The model under review builds one solid part; all positions refer to its coordinate system, in mm. A direction names the side the tool comes from. Round coordinates to 2 decimals unless told otherwise and drop trailing zeros. Loops run counter-clockwise (first coordinate to the right, second up) from the corner with the lowest first, then second, coordinate; pieces in that order, holes last. Notation, with made-up numbers: M 3.25,30 L 55.25,30 A19 cw 55.25,54 Z; hole C 78,-1 d3. An arc over 180 degrees is marked long. Answer in a Markdown table with one row per item. Add a question column.
from build123d import *

# Parameters (mm, degrees)
EXTRUDE_THIN1_DEPTH                       = 20
SKETCH2_R                                 = 20
BOSS_EXTRUDE1_DEPTH                       = 42
FILLET1_RADIUS                            = 20
FILLET1_LENGTH                            = 12
SKETCH3_R                                 = 15
BOSS_EXTRUDE2_DEPTH                       = 21
SKETCH4_R                                 = 11.5
BOSS_EXTRUDE3_DEPTH                       = 10
CUT_EXTRUDE1_START                        = -10
CUT_EXTRUDE1_DEPTH                        = 10
F_18_0_18_DIAMETER_HOLE1_D                = 18
CBORE_FOR_M8_HEX_HEAD_BOLT1_OUTLINE_R     = 4.5
CBORE_FOR_M8_HEX_HEAD_BOLT1_DEPTH         = 43
CBORE_FOR_M8_HEX_HEAD_BOLT1_2_OUTLINE_R   = 9.005
CBORE_FOR_M8_HEX_HEAD_BOLT1_2_OUTLINE_R_2 = 4.5
CBORE_FOR_M8_HEX_HEAD_BOLT1_2_DEPTH       = 5.68
FILLET2_R                                 = 2


# Read off the part's stored shape, not the designer's step: CBORE for M8 Hex Head Bolt1
with BuildPart() as part:
    # Sketch1 → Extrude-Thin1 (new, symmetric)
    with BuildSketch(Plane(origin=(0, 0, 0), x_dir=(0, 0, -1), z_dir=(1, 0, 0))):
        with BuildLine():
            Line((0, 0), (52, 0))
            ThreePointArc((52, 0), (64.727922061, 5.272077939), (70, 18))
            Line((70, 18), (70, 57))
            ThreePointArc((70, 57), (64.727922061, 69.727922061), (52, 75))
            Line((52, 75), (-30, 75))
            Line((-30, 75), (-30, 63))
            Line((-30, 63), (52, 63))
            ThreePointArc((52, 63), (56.242640687, 61.242640687), (58, 57))
            Line((58, 57), (58, 18))
            ThreePointArc((58, 18), (56.242640687, 13.757359313), (52, 12))
            Line((52, 12), (0, 12))
            Line((0, 12), (0, 0))
        make_face()
    extrude(amount=EXTRUDE_THIN1_DEPTH, both=True)

    # Sketch2 → Boss-Extrude1 (add)
    with BuildSketch(Plane.XZ.offset(-63)):
        with Locations(Location((0, 30, 0), (0, 0, 270))):
            Circle(SKETCH2_R)
    extrude(amount=-BOSS_EXTRUDE1_DEPTH)

    # Fillet1: full round fillet: the end face becomes a half cylinder, R = half its width
    fillet1_face = Plane((0, 6, 0), x_dir=(0, -1, 0), z_dir=(0, 0, 1))  # on the end face: x along it, z out of the body
    fillet1_slab = fillet1_face.offset(-FILLET1_RADIUS / 2) * Box(FILLET1_LENGTH, 2 * FILLET1_RADIUS, FILLET1_RADIUS, mode=Mode.PRIVATE)  # the body's end, R deep
    fillet1_round = Plane((0, 6, -20), x_dir=(0, 0, 1), z_dir=(0, -1, 0)) * Cylinder(FILLET1_RADIUS, FILLET1_LENGTH, mode=Mode.PRIVATE)  # its axis R under the face
    add(fillet1_slab - fillet1_round, mode=Mode.SUBTRACT)

    # Sketch3 → Boss-Extrude2 (add)
    with BuildSketch(Plane(origin=(0, 12, 0), x_dir=(1, 0, 0), z_dir=(0, 1, 0))):
        with Locations(Location((0, 20, 0), (0, 0, 90))):
            Circle(SKETCH3_R)
    extrude(amount=BOSS_EXTRUDE2_DEPTH)

    # Sketch4 → Boss-Extrude3 (add)
    with BuildSketch(Plane(origin=(0, 33, 0), x_dir=(1, 0, 0), z_dir=(0, 1, 0))):
        with Locations(Location((0, 20, 0), (0, 0, 90))):
            Circle(SKETCH4_R)
    extrude(amount=BOSS_EXTRUDE3_DEPTH)

    # Sketch5 → Cut-Extrude1 (cut)
    with BuildSketch(Plane(origin=(0, 105, 0), x_dir=(1, 0, 0), z_dir=(0, 1, 0)).offset(CUT_EXTRUDE1_START)):
        with BuildLine():
            Line((-19.078784028, -24), (19.078784028, -24))
            ThreePointArc((19.078784028, -24), (0, -10), (-19.078784028, -24))
        make_face()
        with BuildLine():
            Line((-19.078784028, -36), (19.078784028, -36))
            ThreePointArc((19.078784028, -36), (0, -50), (-19.078784028, -36))
        make_face()
    extrude(amount=CUT_EXTRUDE1_DEPTH, mode=Mode.SUBTRACT)

    # Ø18.0 (18) Diameter Hole1 (through all)
    with Locations(Plane(origin=(0, 63, 0), x_dir=(-1, 0, 0), z_dir=(0, -1, 0))):
        with Locations((0, -30)):
            Hole(F_18_0_18_DIAMETER_HOLE1_D / 2)

    # CBORE for M8 Hex Head Bolt1 outline → CBORE for M8 Hex Head Bolt1 (cut)
    with BuildSketch(Plane(origin=(0, 0, 0), x_dir=(1, 0, 0), z_dir=(0, 1, 0))):
        with Locations((0, 20)):
            Circle(CBORE_FOR_M8_HEX_HEAD_BOLT1_OUTLINE_R)
    extrude(amount=CBORE_FOR_M8_HEX_HEAD_BOLT1_DEPTH, mode=Mode.SUBTRACT)

    # CBORE for M8 Hex Head Bolt1 2 outline → CBORE for M8 Hex Head Bolt1 2 (cut)
    with BuildSketch(Plane(origin=(0, 0, 0), x_dir=(1, 0, 0), z_dir=(0, 1, 0))):
        with Locations((0, 20)):
            Circle(CBORE_FOR_M8_HEX_HEAD_BOLT1_2_OUTLINE_R)
        with Locations((0, 20)):
            Circle(CBORE_FOR_M8_HEX_HEAD_BOLT1_2_OUTLINE_R_2, mode=Mode.SUBTRACT)
    extrude(amount=CBORE_FOR_M8_HEX_HEAD_BOLT1_2_DEPTH, mode=Mode.SUBTRACT)

    # Fillet2
    # the kernel refuses this fillet: 2 mm, written as the material it takes off along each edge
    with BuildSketch(Plane(origin=(20, 63, 30), x_dir=(0, 1, 0), z_dir=(0, 0, -1))) as fillet2_piece_1:
        with BuildLine():
            CenterArc((FILLET2_R, -FILLET2_R), FILLET2_R, 90, 90)
            Line((0, -FILLET2_R), (0, 0))
            Line((0, 0), (FILLET2_R, 0))
        make_face()
    extrude(amount=82, mode=Mode.SUBTRACT)
    with BuildSketch(Plane(origin=(-20, 18, -52), x_dir=(0, 0, -1), z_dir=(0, 1, 0))) as fillet2_piece_2:
        with BuildLine():
            CenterArc((6 + FILLET2_R, -FILLET2_R), FILLET2_R, 90, 90)
            Line((6 + FILLET2_R, 0), (6, 0))
            Line((6, 0), (6, -FILLET2_R))
        make_face()
    revolve(axis=Axis((-20, 18, -52), (-1, 0, 0)), revolution_arc=90, mode=Mode.SUBTRACT)
    with BuildSketch(Plane(origin=(-20, 57, -58), x_dir=(0, 0, -1), z_dir=(0, -1, 0)), Plane(origin=(-20, 18, -70), x_dir=(0, 0, 1), z_dir=(0, 1, 0))) as fillet2_piece_3:
        with BuildLine():
            CenterArc((FILLET2_R, FILLET2_R), FILLET2_R, 180, 90)
            Line((0, FILLET2_R), (0, 0))
            Line((0, 0), (FILLET2_R, 0))
        make_face()
    extrude(amount=39, mode=Mode.SUBTRACT)
    with BuildSketch(Plane(origin=(-20, 57, -52), x_dir=(0, 1, 0), z_dir=(0, 0, 1))) as fillet2_piece_4:
        with BuildLine():
            CenterArc((6 + FILLET2_R, -FILLET2_R), FILLET2_R, 90, 90)
            Line((6, -FILLET2_R), (6, 0))
            Line((6, 0), (6 + FILLET2_R, 0))
        make_face()
    revolve(axis=Axis((-20, 57, -52), (-1, 0, 0)), revolution_arc=90, mode=Mode.SUBTRACT)
    with BuildSketch(Plane(origin=(-20, 63, 30), x_dir=(0, 1, 0), z_dir=(0, 0, -1))) as fillet2_piece_5:
        with BuildLine():
            CenterArc((FILLET2_R, FILLET2_R), FILLET2_R, 180, 90)
            Line((0, FILLET2_R), (0, 0))
            Line((0, 0), (FILLET2_R, 0))
        make_face()
    extrude(amount=82, mode=Mode.SUBTRACT)
    with BuildSketch(Plane(origin=(-20, 75, -52), x_dir=(0, -1, 0), z_dir=(0, 0, 1))) as fillet2_piece_6_section:
        with BuildLine():
            CenterArc((FILLET2_R, FILLET2_R), FILLET2_R, 180, 90)
            Line((0, FILLET2_R), (0, 0))
            Line((0, 0), (FILLET2_R, 0))
        make_face()
    fillet2_piece_6 = extrude(amount=87, mode=Mode.PRIVATE)
    fillet2_piece_6 = fillet2_piece_6 - Plane(origin=(0, 74.534164155, 30), x_dir=(0, 0, -1), z_dir=(0, -1, 0)) * Cylinder(20, 182, mode=Mode.PRIVATE)
    add(fillet2_piece_6, mode=Mode.SUBTRACT)
    with BuildSketch(Plane(origin=(20, 57, -52), x_dir=(0, 1, 0), z_dir=(0, 0, 1))) as fillet2_piece_7:
        with BuildLine():
            CenterArc((6 + FILLET2_R, FILLET2_R), FILLET2_R, 180, 90)
            Line((6, FILLET2_R), (6, 0))
            Line((6, 0), (6 + FILLET2_R, 0))
        make_face()
    revolve(axis=Axis((20, 57, -52), (-1, 0, 0)), revolution_arc=90, mode=Mode.SUBTRACT)
    with BuildSketch(Plane(origin=(20, 57, -58), x_dir=(0, 0, -1), z_dir=(0, -1, 0)), Plane(origin=(20, 18, -70), x_dir=(0, 0, 1), z_dir=(0, 1, 0))) as fillet2_piece_8:
        with BuildLine():
            CenterArc((FILLET2_R, -FILLET2_R), FILLET2_R, 90, 90)
            Line((0, -FILLET2_R), (0, 0))
            Line((0, 0), (FILLET2_R, 0))
        make_face()
    extrude(amount=39, mode=Mode.SUBTRACT)
    with BuildSketch(Plane(origin=(20, 18, -52), x_dir=(0, 0, -1), z_dir=(0, 1, 0))) as fillet2_piece_9:
        with BuildLine():
            CenterArc((6 + FILLET2_R, FILLET2_R), FILLET2_R, 180, 90)
            Line((6 + FILLET2_R, 0), (6, 0))
            Line((6, 0), (6, FILLET2_R))
        make_face()
    revolve(axis=Axis((20, 18, -52), (-1, 0, 0)), revolution_arc=90, mode=Mode.SUBTRACT)
    with BuildSketch(Plane(origin=(20, 18, -52), x_dir=(0, -1, 0), z_dir=(0, 0, 1))) as fillet2_piece_10:
        with BuildLine():
            CenterArc((18 - FILLET2_R, -FILLET2_R), FILLET2_R, 0, 90)
            Line((18, -FILLET2_R), (18, 0))
            Line((18, 0), (18 - FILLET2_R, 0))
        make_face()
    revolve(axis=Axis((20, 18, -52), (1, 0, 0)), revolution_arc=90, mode=Mode.SUBTRACT)
    with BuildSketch(Plane(origin=(0, 63, 30), x_dir=(1, 0, 0), z_dir=(0, 0, -1))) as fillet2_piece_11:
        with BuildLine():
            CenterArc((20 - FILLET2_R, -FILLET2_R), FILLET2_R, 0, 90)
            Line((20, -FILLET2_R), (20, 0))
            Line((20, 0), (20 - FILLET2_R, 0))
        make_face()
    revolve(axis=Axis((0, 63, 30), (0, -1, 0)), revolution_arc=180, mode=Mode.SUBTRACT)
    with BuildSketch(Plane(origin=(20, 57, -52), x_dir=(0, 0, -1), z_dir=(0, -1, 0))) as fillet2_piece_12:
        with BuildLine():
            CenterArc((18 - FILLET2_R, -FILLET2_R), FILLET2_R, 0, 90)
            Line((18, -FILLET2_R), (18, 0))
            Line((18, 0), (18 - FILLET2_R, 0))
        make_face()
    revolve(axis=Axis((20, 57, -52), (1, 0, 0)), revolution_arc=90, mode=Mode.SUBTRACT)
    with BuildSketch(Plane(origin=(20, 12, -52), x_dir=(-1, 0, 0), z_dir=(0, 0, 1)), Plane(origin=(-20, 0, -20), x_dir=(0, 1, 0), z_dir=(0, 0, -1))) as fillet2_piece_13:
        with BuildLine():
            CenterArc((FILLET2_R, FILLET2_R), FILLET2_R, 180, 90)
            Line((0, FILLET2_R), (0, 0))
            Line((0, 0), (FILLET2_R, 0))
        make_face()
    extrude(amount=32, mode=Mode.SUBTRACT)
    with BuildSketch(Plane(origin=(20, 0, -20), x_dir=(0, 1, 0), z_dir=(0, 0, -1)), Plane(origin=(-20, 12, -52), x_dir=(1, 0, 0), z_dir=(0, 0, 1))) as fillet2_piece_14:
        with BuildLine():
            CenterArc((FILLET2_R, -FILLET2_R), FILLET2_R, 90, 90)
            Line((0, -FILLET2_R), (0, 0))
            Line((0, 0), (FILLET2_R, 0))
        make_face()
    extrude(amount=32, mode=Mode.SUBTRACT)
    with BuildSketch(Plane(origin=(20, 75, -52), x_dir=(0, -1, 0), z_dir=(0, 0, 1))) as fillet2_piece_15_section:
        with BuildLine():
            CenterArc((FILLET2_R, -FILLET2_R), FILLET2_R, 90, 90)
            Line((0, -FILLET2_R), (0, 0))
            Line((0, 0), (FILLET2_R, 0))
        make_face()
    fillet2_piece_15 = extrude(amount=87, mode=Mode.PRIVATE)
    fillet2_piece_15 = fillet2_piece_15 - Plane(origin=(0, 74.534164154, 30), x_dir=(0, 0, -1), z_dir=(0, -1, 0)) * Cylinder(20, 182, mode=Mode.PRIVATE)
    add(fillet2_piece_15, mode=Mode.SUBTRACT)
    with BuildSketch(Plane(origin=(0, 12, -20), x_dir=(-1, 0, 0), z_dir=(0, 0, -1))) as fillet2_piece_16:
        with BuildLine():
            CenterArc((20 - FILLET2_R, -FILLET2_R), FILLET2_R, 0, 90)
            Line((20, -FILLET2_R), (20, 0))
            Line((20, 0), (20 - FILLET2_R, 0))
        make_face()
    revolve(axis=Axis((0, 12, -20), (0, 1, 0)), revolution_arc=180, mode=Mode.SUBTRACT)
    with BuildSketch(Plane(origin=(0, 0, -20), x_dir=(-1, 0, 0), z_dir=(0, 0, -1))) as fillet2_piece_17:
        with BuildLine():
            CenterArc((20 - FILLET2_R, FILLET2_R), FILLET2_R, 270, 90)
            Line((20 - FILLET2_R, 0), (20, 0))
            Line((20, 0), (20, FILLET2_R))
        make_face()
    revolve(axis=Axis((0, 0, -20), (0, 1, 0)), revolution_arc=180, mode=Mode.SUBTRACT)
    with BuildSketch(Plane(origin=(-20, 57, -52), x_dir=(0, 0, -1), z_dir=(0, -1, 0))) as fillet2_piece_18:
        with BuildLine():
            CenterArc((18 - FILLET2_R, FILLET2_R), FILLET2_R, 270, 90)
            Line((18, FILLET2_R), (18, 0))
            Line((18, 0), (18 - FILLET2_R, 0))
        make_face()
    revolve(axis=Axis((-20, 57, -52), (1, 0, 0)), revolution_arc=90, mode=Mode.SUBTRACT)
    with BuildSketch(Plane(origin=(-20, 18, -52), x_dir=(0, -1, 0), z_dir=(0, 0, 1))) as fillet2_piece_19:
        with BuildLine():
            CenterArc((18 - FILLET2_R, FILLET2_R), FILLET2_R, 270, 90)
            Line((18, FILLET2_R), (18, 0))
            Line((18, 0), (18 - FILLET2_R, 0))
        make_face()
    revolve(axis=Axis((-20, 18, -52), (1, 0, 0)), revolution_arc=90, mode=Mode.SUBTRACT)


solid = part.part
1. To check wall thickness, follow probe 1 along Y at (x, z) = (16.5, -21); probe 2 along Y at (x, z) = (2, -31); probe 3 along X at (y, z) = (27, -20). State the ranges of each line that lie inside material, in increasing order.
2. For pin 1 Ø1 at (x, z) = (-0.5, -18.5) entering from +Y; pin 2 Ø8 at (x, y) = (-14.5, 98.5) entering from +Z; pin 3 Ø18 at (x, z) = (2.5, 9) entering from -Y; pin 4 Ø20 at (x, z) = (-3, -23.5) entering from -Y, all flat-tipped, find the tip position at first contact; note any pin that passes through.
3. Mouldability with a two-part tool opening along Z and no side actions: class faces 5 (the flat face through (0, 43, -25)), 6 (the cylindrical face through (0.252, 69.587, -64.867)), 7 (the cylindrical face through (0.252, 13.804, -56.289)) as released by +Z, released by -Z, zero draft, split by the parting line, or undercut.
4. Machinability: for faces 1 (the flat face through (9, 33, -28)), 2 (the flat face through (0, 38, -58)), 3 (the cylindrical face through (4.841, 2.8, -27.593)), 4 (the cylindrical face through (0, 6, 0)), which of the approach directions +Z, -Z, +X, -X, +Y, -Y give a long, thin tool a straight path to every point of the face, cutting with its end or side? Answer none if there is none.
5. Take a section at C-C, the plane z = -45. State the section outline as (x, y) points.
6. Take a section at D-D, the plane x = 0. State how many separate pieces and enclosed holes the cut face has, and give its area (3 significant figures).
7. Take a section at B-B, the plane y = 97. State the section outline as (x, z) points, and give its area (3 significant figures).
8. Take a section at A-A, the plane y = 31. State the section outline as (x, z) points.
Check sheet entries:
| question | item | result |
|---|---|---|
| 1 | probe 1 | y = 0 to 12, 63 to 75 |
| 1 | probe 2 | y = 0 to 43, 63 to 75 |
| 1 | probe 3 | x = -15 to -4.5, 4.5 to 15 |
| 2 | pin 1 | stops at y = 75 |
| 2 | pin 2 | stops at z = 45.56 |
| 2 | pin 3 | stops at y = 63 |
| 2 | pin 4 | stops at y = 0 |
| 3 | face 5 | zero draft |
| 3 | face 6 | released by -Z |
| 3 | face 7 | undercut |
| 4 | face 1 | none |
| 4 | face 2 | +X, -X |
| 4 | face 3 | -Y |
| 4 | face 4 | +Z, -Y |
| 5 | outline | M -20,2 A2 ccw -18,0 L 18,0 A2 ccw 20,2 L 20,10 A2 ccw 18,12 L -18,12 A2 ccw -20,10 Z; M -20,65 A2 ccw -18,63 L 18,63 A2 ccw 20,65 L 20,73 A2 ccw 18,75 L -18,75 A2 ccw -20,73 Z |
| 6 | separate pieces | 3 |
| 6 | enclosed holes | 0 |
| 6 | area | 3,410 mm^2 |
| 7 | outline | M -19.08,24 L -6.71,24 A9 cw -6.71,36 L -19.08,36 A20 ccw Z; M 6.71,24 L 19.08,24 A20 ccw 19.08,36 L 6.71,36 A9 cw Z |
| 7 | area | 274 mm^2 |
| 8 | outline | M -20,-68 A2 ccw -18,-70 L 18,-70 A2 ccw 20,-68 L 20,-60 A2 ccw 18,-58 L -18,-58 A2 ccw -20,-60 Z; C 0,-20 d30; hole C 0,-20 d9 |
